from build123d import *

# Parameters (mm, degrees)
SKETCH1_R           = 11.45
BOSS_EXTRUDE1_DEPTH = 7
SKETCH2_R           = 10
BOSS_EXTRUDE2_DEPTH = 4
SKETCH3_R           = 4.7
CUT_EXTRUDE1_DEPTH  = 20.575622595
CHAMFER1_SIZE       = 0.5


with BuildPart() as part:
    # Sketch1 → Boss-Extrude1 (new body)
    with BuildSketch(Plane(origin=(0, 0, 0), x_dir=(0, 0, -1), z_dir=(1, 0, 0))):
        Circle(SKETCH1_R)
    extrude(amount=BOSS_EXTRUDE1_DEPTH)

    # Sketch2 → Boss-Extrude2 (add)
    with BuildSketch(Plane(origin=(7, 0, 0), x_dir=(0, 0, -1), z_dir=(1, 0, 0))):
        Circle(SKETCH2_R)
    extrude(amount=BOSS_EXTRUDE2_DEPTH)

    # Sketch3 → Cut-Extrude1 (cut, through all)
    with BuildSketch(Plane(origin=(11, 0, 0), x_dir=(0, 0, -1), z_dir=(1, 0, 0))):
        Circle(SKETCH3_R)
    extrude(amount=-CUT_EXTRUDE1_DEPTH, mode=Mode.SUBTRACT)

    # Chamfer1
    chamfer1_edges = [part.edges().sort_by_distance(p)[0] for p in [
        (0, 0, 4.7),
        (0, 0, 11.45),
        (11, 0, 10),
    ]]
    chamfer(chamfer1_edges, length=CHAMFER1_SIZE)


solid = part.part
Check sheet for the modelled part. Datum: model origin and axes. Units: mm. A direction names the side the tool comes from. Round coordinates to 2 decimals unless told otherwise and drop trailing zeros. Loops run counter-clockwise (first coordinate to the right, second up) from the corner with the lowest first, then second, coordinate; pieces in that order, holes last. Notation, with made-up numbers: (-30, -35.75) -> (2, -35.75) arc R26 ccw to (2, -2.75) -> close; hole circle Ø3 at (-0.5, -31). An arc over 180 degrees is marked (long way). Put each result on its own line as item: value. Start each with the question number.
1. Scan lines: probe 1 along Y at (x, z) = (4.75, 0); probe 2 along Y at (x, z) = (7.75, 0); probe 3 along Z at (x, y) = (8.25, -0.25). Record each from-to range of solid material in increasing order.
2. Gauge pin test, flat ends, axial feed: pin 1 (1.5 mm diameter, centred on x = 2.5, y = 5.5, fed in from +Z); pin 2 (5 mm diameter, centred on x = 7.5, z = 3.5, fed in from +Y); pin 3 (7.5 mm diameter, centred on y = 0, z = 0, fed in from -X); pin 4 (2 mm diameter, centred on x = 4.5, z = -3.5, fed in from -Y). Record the tip position at first contact, or that the pin passes through.
3. Section check A-A (y = 0). Enter the section's corners in (x, z).
4. Draft check along Z on faces 3 (the face through (5.82, -4.59, 1.02)), 4 (the face through (8.73, -9.76, 2.17)), 5 (the face through (0, -2, -5)). Enter one of: +Z half, -Z half, draft (parallel to the pull), parting line (faces both ways), or undercut.
5. Access from +Z, -Z, +X, -X, +Y, -Y to the whole of each face (thin tool, end or side, straight path). Record for faces 1 (the face through (7, -10.12, -0.79)), 2 (the face through (11, 4.4, 2.2)).
6. Section check D-D (x = 2.75). Enter the section's corners in (y, z), plus the area to 3 significant figures.
7. Section check C-C (x = 9). Enter the section's corners in (y, z), plus the area to 3 significant figures.
Findings:
1. probe 1: y = -11.45 to -4.7, 4.7 to 11.45
1. probe 2: y = -10 to -4.7, 4.7 to 10
1. probe 3: z = -10 to -4.69, 4.69 to 10
2. pin 1: stops at z = 10.42
2. pin 2: stops at y = 11.4
2. pin 3: passes through
2. pin 4: stops at y = -11.17
3. outline: (0, -10.95) -> (0.5, -11.45) -> (7, -11.45) -> (7, -10) -> (10.5, -10) -> (11, -9.5) -> (11, -4.7) -> (0.5, -4.7) -> (0, -5.2) -> close; (0, 5.2) -> (0.5, 4.7) -> (11, 4.7) -> (11, 9.5) -> (10.5, 10) -> (7, 10) -> (7, 11.45) -> (0.5, 11.45) -> (0, 10.95) -> close
4. face 3: undercut
4. face 4: parting line
4. face 5: draft
5. face 1: +X
5. face 2: +Z, -Z, +X, +Y, -Y
6. outline: circle Ø22.9 at (0, 0); hole circle Ø9.4 at (0, 0)
6. area: 342 mm^2
7. outline: circle Ø20 at (0, 0); hole circle Ø9.4 at (0, 0)
7. area: 245 mm^2
